Read the model definition and answer for the solid it produces. Units are mm, in the model's axes. Give positions to 0.01 mm unless a question says otherwise; leave off trailing zeros. Order: outer loops, then holes, each group sorted by start corner. A loop starts at its lowest first (then second) coordinate and runs counter-clockwise, first axis right, second up. Notation, with made-up numbers: M 20.25,86.25 L 72.25,86.25 A15 cw 72.25,98.25 Z; hole C 49.25,80 d6. An arc over 180 degrees is marked long. One line per item, written item: value.
from build123d import *

# Parameters (mm, degrees)
SKETCH_1_R          = 9.5
EXTRUDE_1_DEPTH     = 10
CHAMFER_1_SIZE      = 0.5
CUT_EXTRUDE_2_DEPTH = 10
EXTRUDE_START       = -10
SKETCH_3_R          = 9.5
SKETCH_3_R_2        = 4
EXTRUDE_2_DEPTH     = 10
SKETCH_4_R          = 6
CUT_EXTRUDE_3_DEPTH = 10
SKETCH_5_R          = 6
SKETCH_5_R_2        = 4
EXTRUDE_3_DEPTH     = 10
SKETCH_6_R          = 1.5
CUT_EXTRUDE_4_DEPTH = 244.608292141


with BuildPart() as part:
    # 草图1 → 凸台-拉伸1 (new body)
    with BuildSketch(Plane.XY):
        with BuildLine():
            Line((16.904141504, -9.5), (212.802616478, -9.5))
            Line((212.802616478, -9.5), (215.209800542, -9.5))
            ThreePointArc((215.209800542, -9.5), (219.815462407, -10.037526396), (224.173557789, -11.621212121))
            ThreePointArc((224.173557789, -11.621212121), (243, 0), (224.173557789, 11.621212121))
            ThreePointArc((224.173557789, 11.621212121), (219.815462407, 10.037526396), (215.209800542, 9.5))
            Line((215.209800542, 9.5), (212.802616478, 9.5))
            Line((212.802616478, 9.5), (16.904141504, 9.5))
            ThreePointArc((16.904141504, 9.5), (11.75918395, 10.173090993), (6.960528855, 12.147058824))
            ThreePointArc((6.960528855, 12.147058824), (-14, 0), (6.960528855, -12.147058824))
            ThreePointArc((6.960528855, -12.147058824), (11.75918395, -10.173090993), (16.904141504, -9.5))
        make_face()
        Circle(SKETCH_1_R, mode=Mode.SUBTRACT)
        with Locations((230, 0)):
            Circle(SKETCH_1_R, mode=Mode.SUBTRACT)
    extrude(amount=EXTRUDE_1_DEPTH)

    # 倒角1
    chamfer_1_edges = [part.edges().sort_by_distance(p)[0] for p in [
        (-9.5, 0, 0),
        (-9.5, 0, 10),
    ]]
    chamfer(chamfer_1_edges, length=CHAMFER_1_SIZE)

    # 草图2 → 切除-拉伸2 (cut)
    with BuildSketch(Plane.XY.offset(10)):
        with BuildLine():
            Line((137.499999918, -6), (92.5, -6))
            ThreePointArc((92.5, -6), (86.5, 0), (92.5, 6))
            Line((92.5, 6), (137.499999918, 6))
            ThreePointArc((137.499999918, 6), (143.499999918, 0), (137.499999918, -6))
        make_face()
        with BuildLine():
            Line((35, -6), (72.5, -6))
            ThreePointArc((72.5, -6), (78.5, 0), (72.5, 6))
            Line((72.5, 6), (35, 6))
            ThreePointArc((35, 6), (29, 0), (35, -6))
        make_face()
        with BuildLine():
            Line((157.5, -6), (202.5, -6))
            ThreePointArc((202.5, -6), (208.5, 0), (202.5, 6))
            Line((202.5, 6), (157.5, 6))
            ThreePointArc((157.5, 6), (151.5, 0), (157.5, -6))
        make_face()
    extrude(amount=-CUT_EXTRUDE_2_DEPTH, mode=Mode.SUBTRACT)

    # 草图3 → 凸台-拉伸2 (add)
    with BuildSketch(Plane.XY.offset(10).offset(EXTRUDE_START)):
        with Locations((230, 0)):
            Circle(SKETCH_3_R)
        with Locations((230, 0)):
            Circle(SKETCH_3_R_2, mode=Mode.SUBTRACT)
    extrude(amount=EXTRUDE_2_DEPTH)

    # 草图4 → 切除-拉伸3 (cut)
    with BuildSketch(Plane.XY.offset(10)):
        with Locations((230, 0)):
            Circle(SKETCH_4_R)
    extrude(amount=-CUT_EXTRUDE_3_DEPTH, mode=Mode.SUBTRACT)

    # 草图5 → 凸台-拉伸3 (add)
    with BuildSketch(Plane.XY.offset(10)):
        with Locations((230, 0)):
            Circle(SKETCH_5_R)
        with Locations((230, 0)):
            Circle(SKETCH_5_R_2, mode=Mode.SUBTRACT)
    extrude(amount=-EXTRUDE_3_DEPTH)

    # 草图6 → 切除-拉伸4 (cut, through all)
    with BuildSketch(Plane.XY.offset(10)):
        with Locations((17, 4)):
            Circle(SKETCH_6_R)
        with Locations((17, -4)):
            Circle(SKETCH_6_R)
    extrude(amount=-CUT_EXTRUDE_4_DEPTH, mode=Mode.SUBTRACT)


solid = part.part
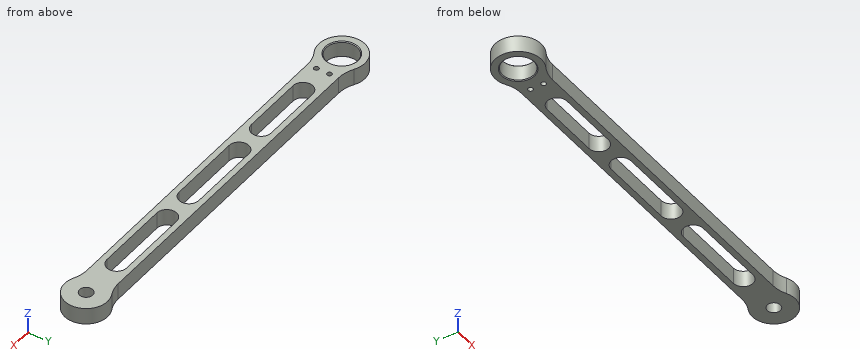
1) Each of these flat-tipped pins is pushed along its axis until it touches: pin 1 Ø5 at (x, z) = (182.5, 2.5) entering from +Y; pin 2 Ø11.5 at (x, y) = (0, 0) entering from +Z; pin 3 Ø3 at (y, z) = (-11, 7.5) entering from +X; pin 4 Ø3 at (y, z) = (8, 2) entering from +X. Where does it stop, or does it pass through?
Reported:
pin 1: stops at y = 9.5
pin 2: passes through
pin 3: stops at x = 238.87
pin 4: stops at x = 241.26
2) Find section C-C, the plane z = 7.5. Write down the section's boundary in (x, y), plus the area to 3 significant figures.
Reported:
outline: M 6.96,-12.15 A20 cw 16.9,-9.5 L 215.21,-9.5 A20 cw 224.17,-11.62 A13 ccw long 224.17,11.62 A20 cw 215.21,9.5 L 16.9,9.5 A20 cw 6.96,12.15 A14 ccw long Z; hole C 0,0 d19; hole C 17,-4 d3; hole C 17,4 d3; hole M 35,-6 L 72.5,-6 A6 ccw 72.5,6 L 35,6 A6 ccw Z; hole M 92.5,-6 L 137.5,-6 A6 ccw 137.5,6 L 92.5,6 A6 ccw Z; hole M 157.5,-6 L 202.5,-6 A6 ccw 202.5,6 L 157.5,6 A6 ccw Z; hole C 230,0 d8
area: 2,850 mm^2
3) Find section A-A, the plane x = 57.5. Write down the section's boundary in (y, z), plus the area to 3 significant figures.
Reported:
outline: M -9.5,0 L -6,0 L -6,10 L -9.5,10 Z; M 6,0 L 9.5,0 L 9.5,10 L 6,10 Z
area: 70.0 mm^2
4) Find section B-B, the plane y = 0. Write down the section's boundary in (x, z).
Reported:
outline: M -14,0 L -10,0 L -9.5,0.5 L -9.5,9.5 L -10,10 L -14,10 Z; M 9.5,0.5 L 10,0 L 29,0 L 29,10 L 10,10 L 9.5,9.5 Z; M 78.5,0 L 86.5,0 L 86.5,10 L 78.5,10 Z; M 143.5,0 L 151.5,0 L 151.5,10 L 143.5,10 Z; M 208.5,0 L 226,0 L 226,10 L 208.5,10 Z; M 234,0 L 243,0 L 243,10 L 234,10 Z
5) Find section D-D, the plane x = 230. Write down the section's boundary in (y, z), plus the area to 3 significant figures.
Reported:
outline: M -13,0 L -4,0 L -4,10 L -13,10 Z; M 4,0 L 13,0 L 13,10 L 4,10 Z
area: 180 mm^2
6) Consider probe 1 along Y at (x, z) = (17, 2.75); probe 2 along Y at (x, z) = (230, 8); probe 3 along Y at (x, z) = (185.5, 4.5). Determine where each line is inside the solid, lowest interval first.
Reported:
probe 1: y = -9.5 to -5.5, -2.5 to 2.5, 5.5 to 9.5
probe 2: y = -13 to -4, 4 to 13
probe 3: y = -9.5 to -6, 6 to 9.5
